```python
from build123d import *

# Parameters (mm, degrees)
F0_W           = 304.8
F0_H           = 203.2
F1_DEPTH       = 25.4
F3_SIZE        = 50.8
F4_W           = 228.6
F4_H           = 25.4
F5_DEPTH       = 25.4
F6_R           = 6.35
F8_D           = 9.525
F8_CBORE_D     = 12.7
F8_CBORE_DEPTH = 12.7
F10_D          = 12.7
F10_DEPTH      = 12.7
F10_TIP        = 3.8154649308


with BuildPart() as f1:
    # F0 (on Top) → F1 (new body)
    with BuildSketch(Plane.XY):
        with Locations((0.9524989873, 1.4589339421)):
            Rectangle(F0_W, F0_H)
    extrude(amount=F1_DEPTH)

    # F3
    f3_edges = [f1.edges().sort_by_distance(p)[0] for p in [
        (-151.447501, 103.058934, 12.7),
        (153.352499, 103.058934, 12.7),
    ]]
    chamfer(f3_edges, length=F3_SIZE)

    # F4 (on face) → F5 (cut)
    with BuildSketch(Plane.XZ.offset(100.1410660579)):
        with Locations((0.9524989873, 12.7)):
            Rectangle(F4_W, F4_H)
    extrude(amount=-F5_DEPTH, mode=Mode.SUBTRACT)

    # F6
    f6_edges = [f1.edges().sort_by_distance(p)[0] for p in [
        (-113.347501, -100.141066, 12.7),
        (-113.347501, -74.741066, 12.7),
        (115.252499, -74.741066, 12.7),
        (115.252499, -100.141066, 12.7),
        (153.352499, -100.141066, 12.7),
        (-151.447501, -100.141066, 12.7),
    ]]
    fillet(f6_edges, radius=F6_R)

    # F8 (through all)
    with Locations(Plane.XY.offset(25.4)):
        with Locations((-132.3975010127, -81.0910660579), (-132.3975010127, -4.8910660579), (134.3024989873, -4.8910660579), (134.3024989873, -81.0910660579)):
            CounterBoreHole(F8_D / 2, F8_CBORE_D / 2, F8_CBORE_DEPTH)

    # F10
    with Locations(Plane.XY.offset(25.4)):
        with Locations((-126.0475010127, 34.0471339421), (127.9524989873, 34.0471339421)):
            Hole(F10_D / 2, depth=F10_DEPTH)
            with Locations((0, 0, -(F10_DEPTH + F10_TIP / 2))):  # 118° drill point
                Cone(0, F10_D / 2, F10_TIP, mode=Mode.SUBTRACT)


solid = f1.part
```
Input: part model. Units: mm. Frame: model coordinates. A direction names the side the tool comes from. Give positions to 0.01 mm unless a question says otherwise; leave off trailing zeros. Write each loop counter-clockwise with the first axis right and the second up, starting at its lowest first coordinate (ties: lowest second). Pieces come first, ordered by that corner, then holes. Notation, with made-up numbers: (47.25, 52) - (64.25, 52) arc R18 cw to (64.25, 72) - close; hole circle Ø10 at (-3, 51.5). An arc over 180 degrees is marked (long way). Write item = value, one per line. Start each with the question number.
1. Ray query, L1, parallel to X at y = -89, z = 18; L2, parallel to Y at x = 46.5, z = 10; L3, parallel to X at y = 31, z = 18.25. Return the intervals inside material, ascending.
2. First-contact query: pin 1 Ø6.5 at (x, y) = (-131, -83) entering from +Z; pin 2 Ø12.5 at (x, z) = (-52.5, 15) entering from -Y. Flat tips, straight axial feed; report the tip coordinate or a pass-through.
3. Section query A-A, the plane z = 17.75. Output: boundary loops of the cut face in (x, y).
4. Access query for faces 1 (the cylindrical face through (113.44, -76.65, 12.88)), 2 (the cylindrical face through (134.296, 34.326, 18.961)), 3 (the cylindrical face through (139.06, -80.88, 6.26)). Directions: +Z, -Z, +X, -X, +Y, -Y. A direction counts if a zero-diameter tool reaches every point of the face in a straight line with its end or side. Return the directions, or none.
5. Section query C-C, the plane y = 60. Output: boundary loops of the cut face in (x, z), then the cut area to 3 significant figures.
6. Mould query, pull axis X, two halves, no side actions, for faces 4 (the flat face through (0, 103.059, 13)), 5 (the cylindrical face through (151.542, -98.232, 12.878)), 6 (the cylindrical face through (-111.438, -76.552, 12.878)). Classes: released by +X, released by -X, zero draft, split by the parting line, or undercut.
7. Section query B-B, the plane x = -9. Output: boundary loops of the cut face in (y, z), then the cut area to 3 significant figures.
Check sheet entries:
q1.L1 = -151.45 to -113.35, 115.25 to 153.35
q1.L2 = -74.74 to 103.06
q1.L3 = -151.45 to -131.62, -120.48 to 122.38, 133.52 to 153.35
q2.pin_1 = 12.7
q2.pin_2 = -74.74
q3.outline = (-151.45, -93.79) arc R6.35 ccw to (-145.1, -100.14) - (-119.7, -100.14) arc R6.35 ccw to (-113.35, -93.79) - (-113.35, -81.09) arc R6.35 cw to (-107, -74.74) - (108.9, -74.74) arc R6.35 cw to (115.25, -81.09) - (115.25, -93.79) arc R6.35 ccw to (121.6, -100.14) - (147, -100.14) arc R6.35 ccw to (153.35, -93.79) - (153.35, 52.26) - (102.55, 103.06) - (-100.65, 103.06) - (-151.45, 52.26) - close; hole circle Ø12.7 at (-132.4, -81.09); hole circle Ø12.7 at (-132.4, -4.89); hole circle Ø12.7 at (-126.05, 34.05); hole circle Ø12.7 at (127.95, 34.05); hole circle Ø12.7 at (134.3, -81.09); hole circle Ø12.7 at (134.3, -4.89)
q4.face_1 = +Z, -Z, -Y
q4.face_2 = +Z
q4.face_3 = +Z, -Z
q5.outline = (-143.71, 0) - (145.61, 0) - (145.61, 25.4) - (-143.71, 25.4) - close
q5.area = 7,350 mm2
q6.face_4 = zero draft
q6.face_5 = released by +X
q6.face_6 = undercut
q7.outline = (-74.74, 0) - (103.06, 0) - (103.06, 25.4) - (-74.74, 25.4) - close
q7.area = 4,520 mm2
